Build history of the part. All positions in model axes, mm. Give positions to 0.01 mm unless a question says otherwise; leave off trailing zeros. Order: outer loops, then holes, each group sorted by start corner. A loop starts at its lowest first (then second) coordinate and runs counter-clockwise, first axis right, second up. Notation, with made-up numbers: (32.25, 62) - (65.25, 62) arc R26 ccw to (65.25, 86) - close; hole circle Ø6 at (-21.5, 46.25). An arc over 180 degrees is marked (long way). Write each question's results on one line, items separated by ' | '. Start each with the question number.
1) Cut at A-A on z = 1039. List the corners of the cut face in (x, y).
2) Drop a flat-ended pin along its axis: pin 1 Ø12 at (x, y) = (14.5, 15) entering from -Z. Give the stop position or say it passes through.
3) Drill centre lines: line 1 along X through (y, z) = (16.5, 120); line 2 along X through (y, z) = (1.9, 12.7). Where is each one in solid material? Low to high. Write a range as from..to.
4) Cut at B-B on x = 12.7. List the corners of the cut face in (y, z).
5) Cut at C-C on y = 15.25. List the corners of the cut face in (x, z), plus the area to 3 significant figures.
from build123d import *

# Parameters (mm, degrees)
SKETCH1_W               = 25.4
SKETCH1_H               = 25.4
SKETCH1_W_2             = 20.32
SKETCH1_H_2             = 20.32
BOSS_EXTRUDE1_DEPTH     = 1155.7
SKETCH2_R               = 6.35
CUT_EXTRUDE1_DEPTH      = 1157.258106999
CUT_EXTRUDE2_DEPTH      = 1157.258106999
CUT_EXTRUDE2_DEPTH_BACK = 1157.258106999
SKETCH3_R               = 6.35


with BuildPart() as part:
    # Sketch1 → Boss-Extrude1 (new body)
    with BuildSketch(Plane.XY):
        with Locations((12.7, 12.7)):
            Rectangle(SKETCH1_W, SKETCH1_H)
        with Locations((12.7, 12.7)):
            Rectangle(SKETCH1_W_2, SKETCH1_H_2, mode=Mode.SUBTRACT)
    extrude(amount=BOSS_EXTRUDE1_DEPTH)

    # Sketch2 → Cut-Extrude1 (cut, through all)
    with BuildSketch(Plane.XZ):
        with Locations(Location((12.7, 12.7, 0), (0, 0, 270))):
            Circle(SKETCH2_R)
    extrude(amount=-CUT_EXTRUDE1_DEPTH, mode=Mode.SUBTRACT)

    # Sketch3 → Cut-Extrude2 (cut, two sides: drawn at the far end of the back side and taken through both)
    with BuildSketch(Plane.XZ.offset(-CUT_EXTRUDE2_DEPTH_BACK)):
        with Locations(Location((12.7, 850.9, 0), (0, 0, 270))):
            Circle(SKETCH3_R)
    extrude(amount=CUT_EXTRUDE2_DEPTH + CUT_EXTRUDE2_DEPTH_BACK, mode=Mode.SUBTRACT)


solid = part.part
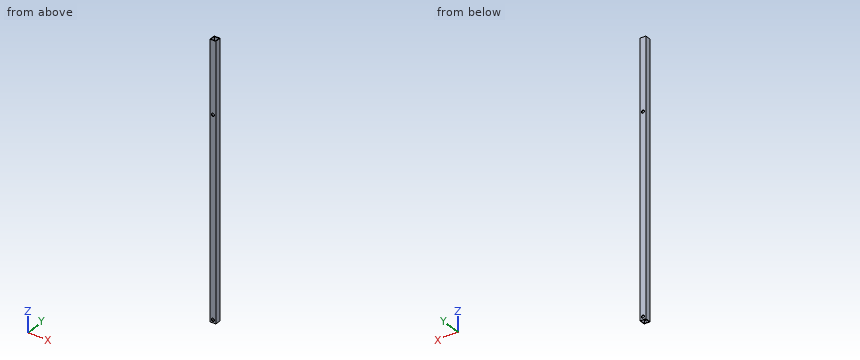
Results:
1) outline: (0, 0) - (25.4, 0) - (25.4, 25.4) - (0, 25.4) - close; hole (2.54, 2.54) - (22.86, 2.54) - (22.86, 22.86) - (2.54, 22.86) - close
2) pin 1: through
3) line 1: 0..2.54, 22.86..25.4 | line 2: 0..6.35, 19.05..25.4
4) outline: (0, 0) - (2.54, 0) - (2.54, 6.35) - (0, 6.35) - close; (0, 19.05) - (2.54, 19.05) - (2.54, 844.55) - (0, 844.55) - close; (0, 857.25) - (2.54, 857.25) - (2.54, 1155.7) - (0, 1155.7) - close; (22.86, 0) - (25.4, 0) - (25.4, 6.35) - (22.86, 6.35) - close; (22.86, 19.05) - (25.4, 19.05) - (25.4, 844.55) - (22.86, 844.55) - close; (22.86, 857.25) - (25.4, 857.25) - (25.4, 1155.7) - (22.86, 1155.7) - close
5) outline: (0, 0) - (2.54, 0) - (2.54, 1155.7) - (0, 1155.7) - close; (22.86, 0) - (25.4, 0) - (25.4, 1155.7) - (22.86, 1155.7) - close | area: 5,870 mm^2
